Design review of the part built by this model. Coordinates are the model's own, in mm. Coordinates: 2 decimals unless noted, no trailing zeros. Loops run counter-clockwise (first coordinate to the right, second up) from the corner with the lowest first, then second, coordinate; pieces in that order, holes last.
Q1. Add section D-D on y = -8. Give the boundary of the cut face in (x, z).
Q2. Draft analysis for pull direction X (two halves, no side actions). For faces 1 (the face through (0, -21, 0)), 2 (the face through (-19.859, 19.797, 0.549)), 3 (the face through (15.266, 17.285, 0.451)), state which applies: released by +X, released by -X, zero draft, split by the parting line, or undercut.
Q3. For P1, Ø2, axis at x = -15.5, y = 15.5, coming from the +Z side, flat-tipped, find the tip position at first contact; note if it passes through.
Q4. Add section A-A on z = -1.75. Give the boundary of the cut face in (x, y), and give its area (3 significant figures).
Q5. Add section B-B on y = -15.5. Give the boundary of the cut face in (x, z).
Q6. Wall thickness on probe 1 along Y at (x, z) = (-15.5, 2.5); probe 2 along X at (y, z) = (0, 0.75): over which ranges is each line inside the solid? List them lowest first.
```python
from build123d import *

# Parameters (mm, degrees)
CYLINDER001_R     = 1.8
CYLINDER001_DEPTH = 20
ARRAY_X_COUNT     = 2
ARRAY_X_PITCH     = 31
ARRAY_Y_COUNT     = 2
ARRAY_Y_PITCH     = 31
CYLINDER_R        = 13
CYLINDER_DEPTH    = 20
BOX_W             = 42
BOX_H             = 42
BOX_DEPTH         = 7
FILLET001_R       = 4


with BuildPart() as motor_attachment_hole_array:
    # Cylinder001 → Cylinder001 (new body)
    with BuildSketch(Plane(origin=(-15.5, -15.5, 0), x_dir=(1, 0, 0), z_dir=(0, 0, 1))):
        Circle(CYLINDER001_R)
    extrude(amount=CYLINDER001_DEPTH)

    # Array X: motor attachment hole array ×2


with BuildPart() as motor_attachment_hole_array_1:
    add(motor_attachment_hole_array.part)
    with Locations(*[(i * ARRAY_X_PITCH, 0, 0) for i in range(1, ARRAY_X_COUNT)]):
        add(motor_attachment_hole_array.part)

    # Array Y: motor attachment hole array ×2


with BuildPart() as motor_attachment_hole_array_2:
    add(motor_attachment_hole_array_1.part)
    with Locations(*[(0, i * ARRAY_Y_PITCH, 0) for i in range(1, ARRAY_Y_COUNT)]):
        add(motor_attachment_hole_array_1.part)


with BuildPart() as fusion001:
    # Cylinder → Cylinder (new body)
    with BuildSketch(Plane.XY):
        Circle(CYLINDER_R)
    extrude(amount=CYLINDER_DEPTH)

    # Fusion001: union motor attachment hole array
    add(motor_attachment_hole_array_2.part)


with BuildPart() as fusion001_1:
    # Fusion001 placement: moved
    add(fusion001.part.moved(Location((0, 0, -5))))


with BuildPart() as motor_side_fillet:
    # Box → Box (new body)
    with BuildSketch(Plane(origin=(-21, -21, -3), x_dir=(1, 0, 0), z_dir=(0, 0, 1))):
        with Locations((21, 21)):
            Rectangle(BOX_W, BOX_H)
    extrude(amount=BOX_DEPTH)

    # Cut002: cut Fusion001
    add(fusion001_1.part, mode=Mode.SUBTRACT)

    # Fillet001
    fillet001_edges = [motor_side_fillet.edges().sort_by_distance(p)[0] for p in [
        (-21, 21, 0.5),
        (21, 21, 0.5),
    ]]
    fillet(fillet001_edges, radius=FILLET001_R)


solid = motor_side_fillet.part
```
Entries:
1. outline: (-21, -3) - (-10.25, -3) - (-10.25, 4) - (-21, 4) - close; (10.25, -3) - (21, -3) - (21, 4) - (10.25, 4) - close
2. face 1: zero draft
2. face 2: released by -X
2. face 3: undercut
3. P1: passes through
4. outline: (-21, -21) - (21, -21) - (21, 17) arc R4 ccw to (17, 21) - (-17, 21) arc R4 ccw to (-21, 17) - close; hole circle Ø3.6 at (-15.5, -15.5); hole circle Ø3.6 at (-15.5, 15.5); hole circle Ø26 at (0, 0); hole circle Ø3.6 at (15.5, -15.5); hole circle Ø3.6 at (15.5, 15.5)
4. area: 1,190 mm2
5. outline: (-21, -3) - (-17.3, -3) - (-17.3, 4) - (-21, 4) - close; (-13.7, -3) - (13.7, -3) - (13.7, 4) - (-13.7, 4) - close; (17.3, -3) - (21, -3) - (21, 4) - (17.3, 4) - close
6. probe 1: y = -21 to -17.3, -13.7 to 13.7, 17.3 to 21
6. probe 2: x = -21 to -13, 13 to 21
